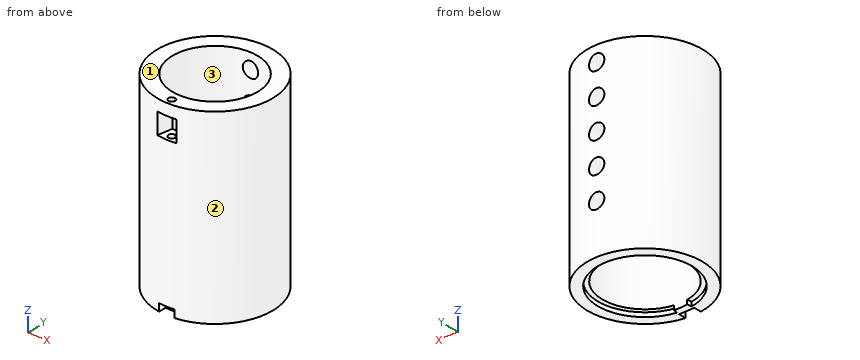
```python
from build123d import *

# Parameters (mm, degrees)
SKETCH1_R           = 15.102178337
SKETCH1_R_2         = 11.15
BOSS_EXTRUDE1_DEPTH = 49
SKETCH2_W           = 2
SKETCH2_H           = 2
CUT_EXTRUDE1_DEPTH  = 2
CUT_EXTRUDE2_DEPTH  = 1.1
SKETCH7_R           = 2
PIN_HOLE_DEPTH      = 54.452329987
CUT_EXTRUDE4_START  = -8.5
CUT_EXTRUDE4_DEPTH  = 5.5
CUT_EXTRUDE5_START  = -15
CUT_EXTRUDE5_DEPTH  = 15


with BuildPart() as part:
    # Sketch1 → Boss-Extrude1 (new body)
    with BuildSketch(Plane.XY):
        Circle(SKETCH1_R)
        Circle(SKETCH1_R_2, mode=Mode.SUBTRACT)
    extrude(amount=BOSS_EXTRUDE1_DEPTH)

    # Sketch2 → Cut-Extrude1 (cut)
    with BuildSketch(Plane(origin=(0, 0, 0), x_dir=(-1, 0, 0), z_dir=(0, 0, -1))):
        with BuildLine():
            Line((2, -14.969161317), (0, -14.969161317))
            Line((0, -14.969161317), (0, -15.102178337))
            ThreePointArc((0, -15.102178337), (1.002209251, -15.068887389), (2, -14.969161317))
        make_face()
        with BuildLine():
            Line((0, -15.102178337), (0, -14.969161317))
            Line((0, -14.969161317), (-2, -14.969161317))
            ThreePointArc((-2, -14.969161317), (-1.002209251, -15.068887389), (0, -15.102178337))
        make_face()
        with Locations((1, -13.969161317)):
            Rectangle(SKETCH2_W, SKETCH2_H)
        with Locations((-1, -13.969161317)):
            Rectangle(SKETCH2_W, SKETCH2_H)
    extrude(amount=-CUT_EXTRUDE1_DEPTH, mode=Mode.SUBTRACT)

    # Sketch6 → Cut-Extrude2 (cut)
    with BuildSketch(Plane(origin=(0, 0, 0), x_dir=(-1, 0, 0), z_dir=(0, 0, -1))):
        with BuildLine():
            Line((-1.931965643, -12.197951006), (-1.744244285, -11.012724998))
            ThreePointArc((-1.744244285, -11.012724998), (-7.241345739, 8.478526516), (11.15, 0))
            ThreePointArc((11.15, 0), (8.478526516, -7.241345739), (1.744244285, -11.012724998))
            Line((1.744244285, -11.012724998), (1.931965643, -12.197951006))
            ThreePointArc((1.931965643, -12.197951006), (9.391013675, -8.020683397), (12.35, 0))
            ThreePointArc((12.35, 0), (-8.020683397, 9.391013675), (-1.931965643, -12.197951006))
        make_face()
    extrude(amount=-CUT_EXTRUDE2_DEPTH, mode=Mode.SUBTRACT)

    # Sketch7 → Pin hole (cut, through all)
    with BuildSketch(Plane(origin=(0, 0, 0), x_dir=(1, 0, 0), z_dir=(0, 1, 0))):
        with Locations(Location((0, -13, 0), (0, 0, 90))):
            Circle(SKETCH7_R)
        with Locations(Location((0, -21, 0), (0, 0, 90))):
            Circle(SKETCH7_R)
        with Locations(Location((0, -29, 0), (0, 0, 90))):
            Circle(SKETCH7_R)
        with Locations(Location((0, -37, 0), (0, 0, 90))):
            Circle(SKETCH7_R)
        with Locations(Location((0, -45, 0), (0, 0, 90))):
            Circle(SKETCH7_R)
    extrude(amount=PIN_HOLE_DEPTH, mode=Mode.SUBTRACT)

    # Sketch8 → Cut-Extrude4 (cut)
    with BuildSketch(Plane.XY.offset(49).offset(CUT_EXTRUDE4_START)):
        with BuildLine():
            Line((2.5, -14.893817192), (1.845760219, -10.996166114))
            ThreePointArc((1.845760219, -10.996166114), (0.926079863, -11.111474974), (0, -11.15))
            Line((0, -11.15), (0, -12.502178337))
            ThreePointArc((0, -12.502178337), (0.636396103, -12.765782234), (0.9, -13.402178337))
            ThreePointArc((0.9, -13.402178337), (0.636396103, -14.038574441), (0, -14.302178337))
            Line((0, -14.302178337), (0, -15.102178337))
            ThreePointArc((0, -15.102178337), (1.254333924, -15.049997905), (2.5, -14.893817192))
        make_face()
        with BuildLine():
            ThreePointArc((0, -11.15), (-0.926079863, -11.111474974), (-1.845760219, -10.996166114))
            Line((-1.845760219, -10.996166114), (-2.5, -14.893817192))
            ThreePointArc((-2.5, -14.893817192), (-1.254333924, -15.049997905), (0, -15.102178337))
            Line((0, -15.102178337), (0, -14.302178337))
            ThreePointArc((0, -14.302178337), (-0.9, -13.402178337), (0, -12.502178337))
            Line((0, -12.502178337), (0, -11.15))
        make_face()
    extrude(amount=CUT_EXTRUDE4_DEPTH, mode=Mode.SUBTRACT)

    # Sketch8<3> → Cut-Extrude5 (cut)
    with BuildSketch(Plane.XY.offset(49).offset(CUT_EXTRUDE5_START)):
        with BuildLine():
            ThreePointArc((0.9, -13.402178337), (0.636396103, -12.765782234), (0, -12.502178337))
            Line((0, -12.502178337), (0, -14.302178337))
            ThreePointArc((0, -14.302178337), (0.636396103, -14.038574441), (0.9, -13.402178337))
        make_face()
        with BuildLine():
            Line((0, -14.302178337), (0, -12.502178337))
            ThreePointArc((0, -12.502178337), (-0.9, -13.402178337), (0, -14.302178337))
        make_face()
    extrude(amount=CUT_EXTRUDE5_DEPTH, mode=Mode.SUBTRACT)


solid = part.part
```
Read the model definition and answer for the solid it produces. Units are mm, in the model's axes. Face numbers are marked on the shaded views. Coordinates: 2 decimals unless noted, no trailing zeros. Loops run counter-clockwise (first coordinate to the right, second up) from the corner with the lowest first, then second, coordinate; pieces in that order, holes last. Notation, with made-up numbers: (24, -39) - (78, -39) arc R25 ccw to (78, -19) - close; hole circle Ø4 at (54.25, 87.5). An arc over 180 degrees is marked (long way). Answer in a Markdown table with one row per item.
1. Determine the mould class of the marked faces 1, 2 and 3 for opening direction Y: +Y half, -Y half, draft (parallel to the pull), parting line (faces both ways), or undercut.
Conclusion:
| item | result |
|---|---|
| face 1 | draft |
| face 2 | parting line |
| face 3 | undercut |
2. Find section C-C, the plane y = 7. Write down the section's boundary in (x, z).
Conclusion:
| item | result |
|---|---|
| outline | (-13.38, 0) - (-10.17, 0) - (-10.17, 1.1) - (-8.68, 1.1) - (-8.68, 49) - (-13.38, 49) - close; (8.68, 1.1) - (10.17, 1.1) - (10.17, 0) - (13.38, 0) - (13.38, 49) - (8.68, 49) - close |
3. Find section B-B, the plane x = 6. Write down the section's boundary in (y, z), then the cut area to 3 significant figures.
Conclusion:
| item | result |
|---|---|
| outline | (-13.86, 0) - (-10.79, 0) - (-10.79, 1.1) - (-9.4, 1.1) - (-9.4, 49) - (-13.86, 49) - close; (9.4, 1.1) - (10.79, 1.1) - (10.79, 0) - (13.86, 0) - (13.86, 49) - (9.4, 49) - close |
| area | 434 mm² |
4. Find section A-A, the plane z = 45. Write down the section's boundary in (x, y).
Conclusion:
| item | result |
|---|---|
| outline | (-2.5, -14.89) - (-1.85, -11) arc R11.15 cw to (-2, 10.97) - (-2, 14.97) arc R15.1 ccw to start; (1.85, -11) - (2.5, -14.89) arc R15.1 ccw to (2, 14.97) - (2, 10.97) arc R11.15 cw to start |
5. Find section D-D, the plane z = 37. Write down the section's boundary in (x, y).
Conclusion:
| item | result |
|---|---|
| outline | (-2, 10.97) - (-2, 14.97) arc R15.1 ccw (long way) to (2, 14.97) - (2, 10.97) arc R11.15 cw (long way) to start; hole circle Ø1.8 at (0, -13.4) |
6. Straight lines are drawn through the part: line 1 (Z direction, x = 1.5, y = -12.5); line 2 (Y direction, x = 0, z = 0.6); line 3 (Y direction, x = 0.5, z = 27.5). For each, find the intervals that lie inside material, in ascending order.
Conclusion:
| item | result |
|---|---|
| line 1 | z = 0 to 40.5, 46 to 49 |
| line 2 | y = -12.97 to -11.15, 12.35 to 15.1 |
| line 3 | y = -15.09 to -11.14 |
7. Given pin 1 (1 mm diameter, centred on x = 7, z = 36, fed in from -Y); pin 2 (6 mm diameter, centred on y = -7.5, z = 42, fed in from +X); pin 3 (8 mm diameter, centred on x = -8, z = 7, fed in from -Y); pin 4 (7.5 mm diameter, centred on x = -4.5, y = 4, fed in from -Z), each flat-ended and moving along its own axis, determine where each tip first touches the part or whether it passes through.
Conclusion:
| item | result |
|---|---|
| pin 1 | stops at y = -13.63 |
| pin 2 | stops at x = 14.42 |
| pin 3 | stops at y = -14.56 |
| pin 4 | passes through |
